Could you check a few things on this model? Use its own coordinates, in mm. A direction names the side the tool comes from. Give positions to 0.01 mm unless a question says otherwise; leave off trailing zeros. Loops run counter-clockwise (first coordinate to the right, second up) from the corner with the lowest first, then second, coordinate; pieces in that order, holes last. Notation, with made-up numbers: M 83,-39.5 L 124,-39.5 A28 cw 124,-9.5 Z; hole C 87,0 d10. An arc over 180 degrees is marked long. Use a Markdown table: item, result. Add a question column.
1) Suppose I cut it at B-B on z = 5.75. List the corners of the cut face in (x, y) for me, and give its area (3 significant figures).
2) Which directions (+Z, -Z, +X, -X, +Y, -Y) give clear straight access to the entire face, cutting with the end or side of a thin tool? Please do faces 4 (the cylindrical face through (-11.2, 6.6, 4.9)), 5 (the flat face through (6, 6, 0)).
3) We'd pull the mould along X, two halves only. Please class faces 1 (the cylindrical face through (4.822, -0.738, -4.33)), 2 (the cylindrical face through (5.5, -5.1, -4.2)), 3 (the cylindrical face through (7.528, -12.974, 4.93)): +X half, -X half, draft (parallel to the pull), parting line (faces both ways), or undercut.
4) If I drill on line 1 along Y through (x, z) = (0, 1); line 2 along X through (y, z) = (0, 1.75); line 3 along Y through (x, z) = (0, -1), over which ranges is the centre line in solid material (lowest first)? Write a range as [from, to].
5) Suppose I cut it at D-D on x = 11.75. List the corners of the cut face in (y, z) for me, and give its area (3 significant figures).
6) Suppose I cut it at A-A on x = 0. List the corners of the cut face in (y, z) for me.
7) Suppose I cut it at C-C on y = 10.75. List the corners of the cut face in (x, z) for me.
8) Will these pins go through, and if not, where does the flat tip stop? pin 1 Ø8 at (y, z) = (-5.5, -5.5) entering from +X; pin 2 Ø6 at (y, z) = (-6.5, 1) entering from -X; pin 3 Ø1 at (y, z) = (6.5, 5) entering from -X.
Autodesk Inventor part; units mm, degrees
ref_plane "Arbeitsebene2" through (-5.3852, -14, 0) normal (0.8825, -0.4703, 0) x (0.4703, 0.8825, 0)
ref_plane "YZ Plane" through (0, 0, 0) normal (1, 0, 0) x (0, 1, 0)
ref_plane "XZ Plane" through (0, 0, 0) normal (0, 1, 0) x (-1, 0, 0)
sketch "Skizze1" plane through (0, 0, 0) normal (0, 0, 1) x (1, 0, 0)
  circle A0 centre (0, 0) radius 15
  line L0 (0, 15) -> (0, -15) construction
  arc A1 (-5.3852, 14) -> (5.3852, 14) centre (0, 28) ccw
  point P0 (0, 0)
  point P1 (0, 13)
  dimension "d0" = 30
  dimension "d1" = 15
  dimension "d2" = 13
extrude "Extrusion1" add sketch "Skizze1" along normal blind 10
extrude "Extrusion2" cut sketch "Skizze1" along normal blind 10 contours A1 A0 picked at (0.6105, 13.7041)
pattern_circular "Runde Anordnung1" count 6 over 360 about axis through (0, 0, 0) along (0, 0, 1) of "Extrusion2"
sketch "Skizze2" plane through (0, 0, 0) normal (0, 0, -1) x (-1, 0, 0)
  circle A0 centre (0, 0) radius 7.5
  dimension "d10" = 15
extrude "Extrusion3" add sketch "Skizze2" along normal blind 10
chamfer "Fasen1" distance 1.5 angle 45 1 edges at (7.5, 0, -10)
sketch "Skizze3" plane through (0, 0, 10) normal (0, 0, 1) x (1, 0, 0)
  circle A0 centre (0, 0) radius 2.5
  dimension "d16" = 5
extrude "Extrusion4" cut sketch "Skizze3" against normal up to surface (20 mm away)
ref_plane "Arbeitsebene2" through (-5.3852, -14, 0) normal (0.8825, -0.4703, 0) x (0.4703, 0.8825, 0)
sketch "Skizze5" plane through (-5.3852, -14, 0) normal (0.8825, -0.4703, 0) x (0.4703, 0.8825, 0)
  circle A0 centre (14.8877, -5) radius 1.75
  point P0 (14.8877, 0)
  dimension "d21" = 3.5
  dimension "d22" = 5
extrude "Extrusion5" cut sketch "Skizze5" along normal through all both and the other way through all
thread "Gewinde2"
thread "Gewinde3"
properties part number "bolt" material "Stahl, galvanisiert"
Answer block:
| question | item | result |
|---|---|---|
| 1 | outline | M -14.82,-2.34 A15 cw -9.43,-11.66 A15 ccw -5.39,-14 A15 cw 5.39,-14 A15 ccw 9.43,-11.66 A15 cw 14.82,-2.34 A15 ccw 14.82,2.34 A15 cw 9.43,11.66 A15 ccw 5.39,14 A15 cw -5.39,14 A15 ccw -9.43,11.66 A15 cw -14.82,2.34 A15 ccw Z; hole C 0,0 d5 |
| 1 | area | 600 mm^2 |
| 2 | face 4 | +Z, -Z, -X, +Y |
| 2 | face 5 | -Z |
| 3 | face 1 | undercut |
| 3 | face 2 | parting line |
| 3 | face 3 | +X half |
| 4 | line 1 | y = [-13, -2.5], [2.5, 13] |
| 4 | line 2 | x = [-15, -2.5], [2.5, 15] |
| 4 | line 3 | y = [-7.5, -2.5], [2.5, 7.5] |
| 5 | outline | M -5.71,0 L 5.71,0 L 5.71,10 L -5.71,10 Z |
| 5 | area | 114 mm^2 |
| 6 | outline | M -13,0 L -7.5,0 L -7.5,-8.5 L -6,-10 L -2.5,-10 L -2.5,10 L -13,10 Z; M 2.5,-10 L 6,-10 L 7.5,-8.5 L 7.5,0 L 13,0 L 13,10 L 2.5,10 Z |
| 7 | outline | M -9.61,0 L 9.61,0 L 9.61,10 L -9.61,10 Z |
| 8 | pin 1 | stops at x = 7.35 |
| 8 | pin 2 | stops at x = -13.54 |
| 8 | pin 3 | stops at x = -11.56 |
